```python
from build123d import *

# Parameters (mm, degrees)
SKETCH_1_W          = 65
SKETCH_1_H          = 45
EXTRUDE_1_DEPTH     = 1.2
FILLET_1_R          = 2
SKETCH_2_5_R        = 3
EXTRUDE_2_DEPTH     = 1.2
SKETCH_2_R          = 1.05
CUT_EXTRUDE_1_DEPTH = 2.2
FILLET_2_R          = 2
SKETCH_3_W          = 18.5
SKETCH_3_H          = 6.5
CUT_EXTRUDE_2_DEPTH = 2.2


with BuildPart() as part:
    # 草图1 → 凸台-拉伸1 (new body)
    with BuildSketch(Plane(origin=(0, 0, 0), x_dir=(1, 0, 0), z_dir=(0, 1, 0))):
        with Locations((32.5, 22.5)):
            Rectangle(SKETCH_1_W, SKETCH_1_H)
    extrude(amount=EXTRUDE_1_DEPTH)

    # 圆角1
    fillet_1_edges = [part.edges().sort_by_distance(p)[0] for p in [
        (0, 0.6, -45),
        (65, 0.6, -45),
        (65, 0.6, 0),
        (0, 0.6, 0),
    ]]
    fillet(fillet_1_edges, radius=FILLET_1_R)

    # 草图2<5> → 凸台-拉伸2 (add)
    with BuildSketch(Plane(origin=(0, 1.2, 0), x_dir=(1, 0, 0), z_dir=(0, 1, 0))):
        with Locations((63, 31)):
            Circle(SKETCH_2_5_R)
        with Locations((2, 27)):
            Circle(SKETCH_2_5_R)
    extrude(amount=-EXTRUDE_2_DEPTH)

    # 草图2 → 切除-拉伸1 (cut, through all)
    with BuildSketch(Plane(origin=(0, 1.2, 0), x_dir=(1, 0, 0), z_dir=(0, 1, 0))):
        with Locations((63, 31)):
            Circle(SKETCH_2_R)
        with Locations((2, 27)):
            Circle(SKETCH_2_R)
    extrude(amount=-CUT_EXTRUDE_1_DEPTH, mode=Mode.SUBTRACT)

    # 圆角2
    fillet_2_edges = [part.edges().sort_by_distance(p)[0] for p in [
        (0, 0.6, -29.236067977),
        (0, 0.6, -24.763932023),
        (65, 0.6, -28.763932023),
        (65, 0.6, -33.236067977),
    ]]
    fillet(fillet_2_edges, radius=FILLET_2_R)

    # 草图3 → 切除-拉伸2 (cut, through all)
    with BuildSketch(Plane(origin=(0, 1.2, 0), x_dir=(1, 0, 0), z_dir=(0, 1, 0))):
        with Locations((52.75, 3.25)):
            Rectangle(SKETCH_3_W, SKETCH_3_H)
    extrude(amount=-CUT_EXTRUDE_2_DEPTH, mode=Mode.SUBTRACT)


solid = part.part
```
Source: CAD feature listing. Evaluate the final solid. Frame: model axes, mm. Round coordinates to 2 decimals unless told otherwise and drop trailing zeros. Loops run counter-clockwise (first coordinate to the right, second up) from the corner with the lowest first, then second, coordinate; pieces in that order, holes last.
1. Ray query, L1, parallel to X at y = 0.8, z = -31; L2, parallel to Z at x = 2, y = 0.45; L3, parallel to Z at x = 63, y = 0.75. Return the intervals inside material, ascending.
2. Section query D-D on z = -35.5. Output: boundary loops of the cut face in (x, y), and give its area (3 significant figures).
3. Contact query for flat-ended pins moving along their axis: pin 1 (0.6 mm diameter, centred on y = 0.5, z = -2.5, fed in from +X); pin 2 (0.6 mm diameter, centred on y = 0.5, z = -3.5, fed in from -X). Output: stop coordinate, or through.
4. Mould query, pull axis Z, two halves, no side actions, for faces 1 (the cylindrical face through (64.4, 0.61, -0.57)), 2 (the flat face through (32, 0, -23)), 3 (the cylindrical face through (63.97, 0.61, -30.6)). Classes: released by +Z, released by -Z, zero draft, split by the parting line, or undercut.
5. Section query B-B on y = 0.6. Output: boundary loops of the cut face in (x, z).
6. Section query C-C on z = -4.5. Output: boundary loops of the cut face in (x, y).
7. Section query A-A on z = -27. Output: boundary loops of the cut face in (x, y).
Answers below:
1. L1: x = 0 to 61.95, 64.05 to 66
1. L2: z = -45 to -28.05, -25.95 to 0
1. L3: z = -45 to -32.05, -29.95 to 0
2. outline: (0, 0) - (65, 0) - (65, 1.2) - (0, 1.2) - close
2. area: 78.0 mm2
3. pin 1: stops at x = 65
3. pin 2: stops at x = 0
4. face 1: released by +Z
4. face 2: zero draft
4. face 3: undercut
5. outline: (-0.4, -28.8) arc R2 cw to (0, -30) - (0, -43) arc R2 ccw to (2, -45) - (63, -45) arc R2 ccw to (65, -43) - (65, -34) arc R2 cw to (65.4, -32.8) arc R3 ccw to (65.4, -29.2) arc R2 cw to (65, -28) - (65, -2) arc R2 ccw to (63, 0) - (62, 0) - (62, -6.5) - (43.5, -6.5) - (43.5, 0) - (2, 0) arc R2 ccw to (0, -2) - (0, -24) arc R2 cw to (-0.4, -25.2) arc R3 ccw to start; hole circle Ø2.1 at (2, -27); hole circle Ø2.1 at (63, -31)
6. outline: (0, 0) - (43.5, 0) - (43.5, 1.2) - (0, 1.2) - close; (62, 0) - (65, 0) - (65, 1.2) - (62, 1.2) - close
7. outline: (-1, 0) - (0.95, 0) - (0.95, 1.2) - (-1, 1.2) - close; (3.05, 0) - (65, 0) - (65, 1.2) - (3.05, 1.2) - close
